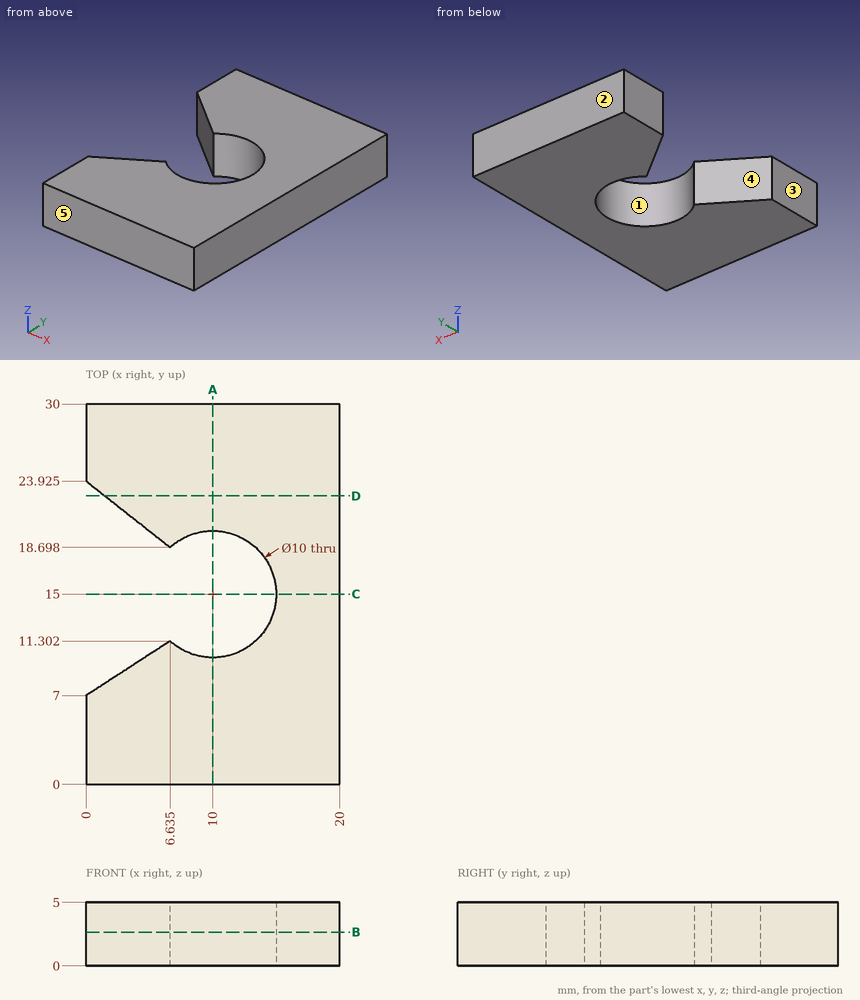
Print and shaded views of the part. All mm, measured from the part's lowest x, y and z. A direction names the side the tool comes from. Coordinates: 2 decimals unless noted, no trailing zeros. Order: outer loops, then holes, each group sorted by start corner. A loop starts at its lowest first (then second) coordinate and runs counter-clockwise, first axis right, second up. Notation, with made-up numbers: (83.25, 50.5) - (139.25, 50.5) arc R7 ccw to (139.25, 58.5) - close; hole circle Ø3 at (55, 73). An arc over 180 degrees is marked (long way). Return JSON: item names as keys, results as strings. Group by question number.
Item 1: Cut at D-D (y = 22.75). List the corners of the cut face in (x, z).
Item 2: Which spindle directions (+Z, -Z, +X, -X, +Y, -Y) get a long thin tool onto all of the face, cutting with end or side? Do the marked faces 4 and 5. Say none if no direction does.
Item 3: Drill centre lines: probe 1 along Y at (x, z) = (10, 2.4); probe 2 along X at (y, z) = (15, 2.6); probe 3 along Y at (x, z) = (8.5, 0.3). Where is each one in solid material? Low to high. Write a range as from..to.
Item 4: Cut at C-C (y = 15). List the corners of the cut face in (x, z), plus the area to 3 significant figures.
Item 5: Pull direction Y, two halves, no side cores. Call the marked faces 1, 2 and 3: pulls with the +Y half, pulls with the -Y half, needs draft (parallel to the pull), parting line crosses it, or undercut.
Item 6: Cut at A-A (x = 10). List the corners of the cut face in (y, z).
Item 7: Cut at B-B (z = 2.65). List the corners of the cut face in (x, y) (1 decimal).
Check values:
{
 "1": {"outline": "(1.49, 0) - (20, 0) - (20, 5) - (1.49, 5) - close"},
 "2": {"face 4": "+Z, -Z, -X", "face 5": "+Z, -Z, +X, -X, -Y"},
 "3": {"probe 1": "y = 0..10, 20..30", "probe 2": "x = 15..20", "probe 3": "y = 0..10.23, 19.77..30"},
 "4": {"outline": "(15, 0) - (20, 0) - (20, 5) - (15, 5) - close", "area": "25.0 mm2"},
 "5": {"face 1": "undercut", "face 2": "pulls with the +Y half", "face 3": "needs draft"},
 "6": {"outline": "(0, 0) - (10, 0) - (10, 5) - (0, 5) - close; (20, 0) - (30, 0) - (30, 5) - (20, 5) - close"},
 "7": {"outline": "(0, 0) - (20, 0) - (20, 30) - (0, 30) - (0, 23.9) - (6.6, 18.7) arc R5 cw (long way) to (6.6, 11.3) - (0, 7) - close"}
}
